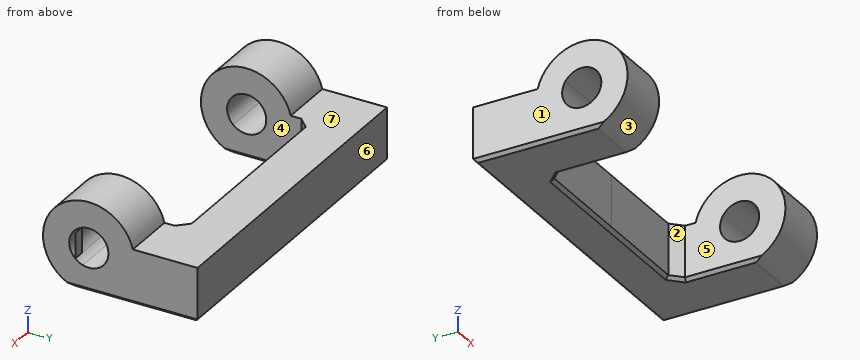
from build123d import *

# Parameters (mm, degrees)
BOSS_EXTRUDE1_DEPTH = 5
CUT_EXTRUDE1_DEPTH  = 31.003999108
SKETCH2_3_R         = 1.799674582
BOSS_EXTRUDE2_DEPTH = 5
SKETCH3_R           = 1.799674582
BOSS_EXTRUDE3_DEPTH = 5
CHAMFER1_SIZE       = 0.3
FILLET1_R           = 0.4


with BuildPart() as part:
    # Model → Boss-Extrude1 (new body)
    with BuildSketch(Plane.XY):
        Polygon((294.639989597, 34.266605248), (295.614474597, 35.240900181), (304.640051213, 35.240024382), (313.667685024, 35.239144856), (314.643988705, 34.264659856), (314.643988705, 28.018126256), (319.643988705, 28.016541689), (319.643988705, 39.239445651), (289.639989597, 39.239424468), (289.639989597, 28.016886869), (294.639989597, 28.020075702), align=None)
    extrude(amount=BOSS_EXTRUDE1_DEPTH)

    # Sketch2 → Cut-Extrude1 (cut, through all)
    with BuildSketch(Plane.ZY.offset(-289.639989597)):
        with BuildLine():
            ThreePointArc((5, 30.738550482), (2.616874768, 30.420409758), (2.676683755, 28.016886869))
            Line((2.676683755, 28.016886869), (5, 28.016886869))
            Line((5, 28.016886869), (5, 30.738550482))
        make_face()
    extrude(amount=-CUT_EXTRUDE1_DEPTH, mode=Mode.SUBTRACT)

    # Sketch2<3> → Boss-Extrude2 (add)
    with BuildSketch(Plane.ZY.offset(-289.639989597)):
        with BuildLine():
            Line((0, 30.526457448), (0, 27.942741433))
            ThreePointArc((0, 27.942741433), (8.175740848, 29.23459944), (0, 30.526457448))
        make_face()
        with Locations((3.985657063, 29.251964795)):
            Circle(SKETCH2_3_R, mode=Mode.SUBTRACT)
    extrude(amount=-BOSS_EXTRUDE2_DEPTH)

    # Sketch3 → Boss-Extrude3 (add)
    with BuildSketch(Plane.ZY.offset(-314.643988705)):
        with BuildLine():
            Line((4.35e-07, 30.526456106), (4.35e-07, 27.942740092))
            ThreePointArc((4.35e-07, 27.942740092), (8.175741283, 29.234598099), (4.35e-07, 30.526456106))
        make_face()
        with Locations((3.985657498, 29.251963453)):
            Circle(SKETCH3_R, mode=Mode.SUBTRACT)
    extrude(amount=-BOSS_EXTRUDE3_DEPTH)

    # Chamfer1
    chamfer1_edges = [part.edges().sort_by_distance(p)[0] for p in [
        (294.639989597, 31.104673341, 0),
        (289.639989597, 33.59108295, 0),
        (304.641989151, 39.239435059, 0),
        (319.643988705, 33.62799367, 0),
        (314.643988705, 31.141393056, 0),
        (314.155836865, 34.751902356, 0),
        (309.153868118, 35.239584619, 0),
        (300.127262905, 35.240462282, 0),
        (295.127232097, 34.753752715, 0),
    ]]
    chamfer(chamfer1_edges, length=CHAMFER1_SIZE)

    # Fillet1
    fillet1_edges = [part.edges().sort_by_distance(p)[0] for p in [
        (317.143988705, 27.942740092, 4.35e-07),
        (292.139989597, 27.942741433, 0),
    ]]
    fillet(fillet1_edges, radius=FILLET1_R)


solid = part.part
Verification items for the finished model (mm, model axes). Face numbers are marked on the shaded views. A direction names the side the tool comes from. Give positions to 0.01 mm unless a question says otherwise; leave off trailing zeros. Write each loop counter-clockwise with the first axis right and the second up, starting at its lowest first coordinate (ties: lowest second). Pieces come first, ordered by that corner, then holes. Notation, with made-up numbers: M -37.75,29.25 L 11.25,29.25 A11 cw 11.25,49.25 Z; hole C 88.25,82.5 d5. An arc over 180 degrees is marked long. Write item = value, one per line.
(1) Sectioned sample at D-D (z = 4). Give the number of separate pieces and of enclosed holes in the cut face, then the cut area to 3 significant figures.
Found:
separate_pieces = 4
enclosed_holes = 0
area = 187 mm2
(2) Sectioned sample at A-A (y = 32.5). Record the cut outline in (x, z).
Found:
outline = M 289.64,0.3 L 289.94,0 L 294.34,0 L 294.64,0.3 L 294.64,6.61 L 289.64,6.61 Z; M 314.64,0.3 L 314.94,0 L 319.34,0 L 319.64,0.3 L 319.64,6.61 L 314.64,6.61 Z
(3) Material ranges on line 1 (X direction, y = 30.5, z = 5.5); line 2 (Y direction, x = 300.5, z = 1); line 3 (Z direction, x = 293, y = 35.5), recorded low to high.
Found:
line_1 = 289.64 to 294.64, 314.64 to 319.64
line_2 = 35.24 to 39.24
line_3 = 0 to 5
(4) Draft check along X on the marked faces 1, 2, 3 and 4. Enter one of: released by +X, released by -X, zero draft, split by the parting line, or undercut.
Found:
face_1 = released by -X
face_2 = undercut
face_3 = zero draft
face_4 = undercut
(5) Go/stop test with flat-tipped pins: pin 1 Ø4 at (x, z) = (310.5, 2) entering from -Y; pin 2 Ø3 at (x, z) = (304.5, 5.5) entering from +Y; pin 3 Ø1.8 at (x, y) = (302, 36.5) entering from +Z. Record where each tip stops, or that it passes through.
Found:
pin_1 = 35.24
pin_2 = 39.24
pin_3 = 5
(6) Access from +Z, -Z, +X, -X, +Y, -Y to the whole of each face (thin tool, end or side, straight path). Record for the marked faces 5, 6 and 7.
Found:
face_5 = +Z, -Z, -Y
face_6 = +Z, -Z, +X, -X, +Y
face_7 = +Z, +X, -X, +Y
(7) Sectioned sample at B-B (z = 6.75). Record the cut outline in (x, y).
Found:
outline = M 289.64,26.09 L 294.64,26.09 L 294.64,32.38 L 289.64,32.38 Z; M 314.64,26.09 L 319.64,26.09 L 319.64,32.38 L 314.64,32.38 Z
